The drawing under review shows one solid part. Ordinate dimensions are in mm from its lowest x, y, z. A direction names the side the tool comes from. Give positions to 0.01 mm unless a question says otherwise; leave off trailing zeros. Loops run counter-clockwise (first coordinate to the right, second up) from the corner with the lowest first, then second, coordinate; pieces in that order, holes last. Notation, with made-up numbers: M 10.5,30 L 68.5,30 A23 cw 68.5,59 Z; hole C 76,-36.5 d4. An arc over 180 degrees is marked long. Put each result on its own line as item: value. Start each with the question number.
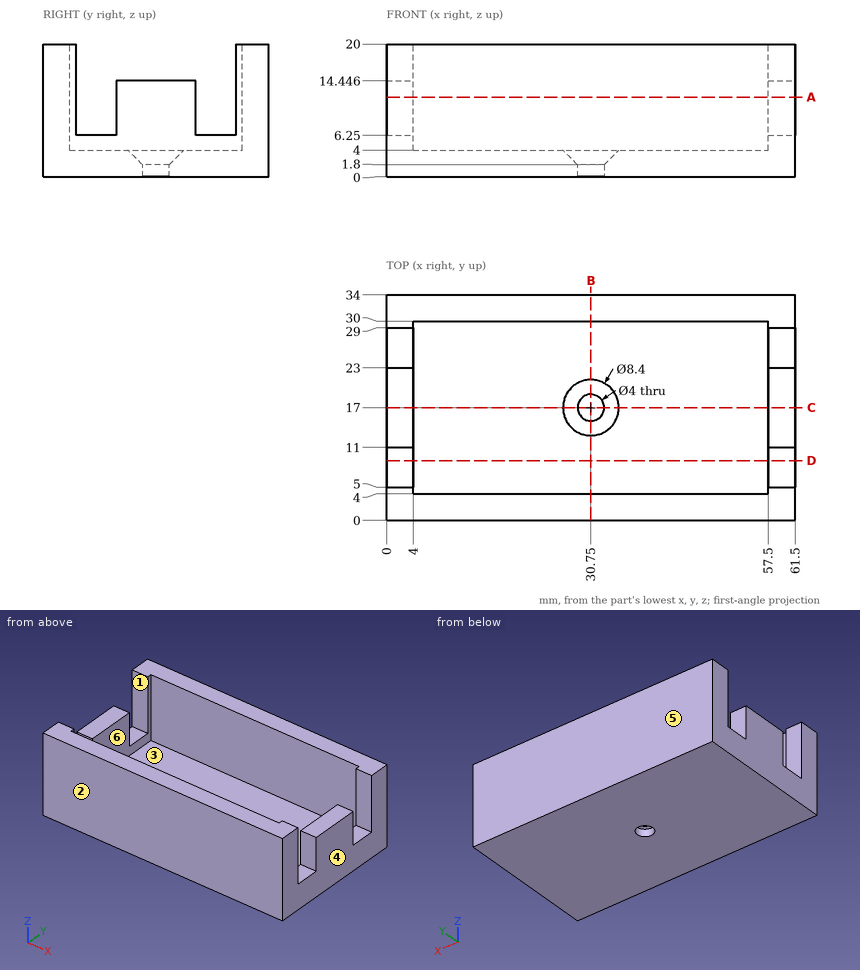
Item 1: Consider section D-D, the plane y = 9. Write out the cut boundary in (x, z).
Item 2: Tool access review of the marked faces 1, 2 and 3: name each direction out of +Z, -Z, +X, -X, +Y, -Y from which nothing blocks a thin tool from reaching the whole face with its end or side.
Item 3: Draft analysis for pull direction X (two halves, no side actions). For the marked faces 4, 5 and 6, state which applies: +X half, -X half, draft (parallel to the pull), parting line (faces both ways), or undercut.
Item 4: Consider section A-A, the plane z = 12. Write out the cut boundary in (x, y).
Item 5: Consider section B-B, the plane x = 30.75. Write out the cut boundary in (y, z).
Item 6: Consider section C-C, the plane y = 17. Write out the cut boundary in (x, z).
Item 7: Clearance check with flat-ended pins moving along their axes: pin 1 Ø3 at (x, z) = (60.5, 10) entering from -Y; pin 2 Ø13 at (x, y) = (36, 14.5) entering from +Z; pin 3 Ø3 at (x, y) = (59, 7.5) entering from +Z; pin 4 Ø4.5 at (x, y) = (59.5, 19.5) entering from +Z. State where each tip first meets the part, or that it passes through.
Item 8: To check wall thickness, follow L1, parallel to Y at x = 49, z = 6; L2, parallel to Y at x = 30.75, z = 0.85; L3, parallel to X at y = 18.5, z = 6. State the ranges of each line that lie inside material, in increasing order. Write a range as [from, to].
Report:
1. outline: M 0,0 L 61.5,0 L 61.5,6.25 L 57.5,6.25 L 57.5,4 L 4,4 L 4,6.25 L 0,6.25 Z
2. face 1: +Z, +X, -X
2. face 2: +Z, -Z, +X, -X, -Y
2. face 3: +Z
3. face 4: +X half
3. face 5: draft
3. face 6: undercut
4. outline: M 0,0 L 61.5,0 L 61.5,5 L 57.5,5 L 57.5,4 L 4,4 L 4,5 L 0,5 Z; M 0,11 L 4,11 L 4,23 L 0,23 Z; M 0,29 L 4,29 L 4,30 L 57.5,30 L 57.5,29 L 61.5,29 L 61.5,34 L 0,34 Z; M 57.5,11 L 61.5,11 L 61.5,23 L 57.5,23 Z
5. outline: M 0,0 L 15,0 L 15,1.8 L 12.8,4 L 4,4 L 4,20 L 0,20 Z; M 19,0 L 34,0 L 34,20 L 30,20 L 30,4 L 21.2,4 L 19,1.8 Z
6. outline: M 0,0 L 28.75,0 L 28.75,1.8 L 26.55,4 L 4,4 L 4,14.45 L 0,14.45 Z; M 32.75,0 L 61.5,0 L 61.5,14.45 L 57.5,14.45 L 57.5,4 L 34.95,4 L 32.75,1.8 Z
7. pin 1: y = 0
7. pin 2: z = 4
7. pin 3: z = 6.25
7. pin 4: z = 14.45
8. L1: [0, 4], [30, 34]
8. L2: [0, 15], [19, 34]
8. L3: [0, 4], [57.5, 61.5]
